Part model, mm, in its own coordinate system. Face numbers are marked on the shaded views. A direction names the side the tool comes from. Round coordinates to 2 decimals unless told otherwise and drop trailing zeros. Write each loop counter-clockwise with the first axis right and the second up, starting at its lowest first coordinate (ties: lowest second). Pieces come first, ordered by that corner, then holes. Notation, with made-up numbers: M -30.5,-37.75 L -10.5,-37.75 A22 cw -10.5,-30.75 Z; hole C 40.5,67.5 d1. An arc over 180 degrees is marked long. One line per question, with ' | ' between items. Start each with the question number.
1) Saw through at B-B (x = 0). Give the number of separate pieces and of enclosed holes in the cut face, plus the area to 3 significant figures.
2) Saw through at D-D (z = 42). List the corners of the cut face in (x, y), plus the area to 3 significant figures.
3) Saw through at A-A (y = 0). List the corners of the cut face in (x, z).
4) Saw through at C-C (z = 53). List the corners of the cut face in (x, y), plus the area to 3 significant figures.
5) Wall check: probe 1 along X at (y, z) = (-28.5, 4.5); probe 2 along X at (y, z) = (-46, 27); probe 3 along X at (y, z) = (-29, 16.5). Give the ranges that are in metal, low to high. Write a range as [from, to].
6) Mould opens along Y. For the marked faces 4, 5 and 6 say: pulls with the +Y half, pulls with the -Y half, needs draft (parallel to the pull), parting line crosses it, or undercut.
7) Tool access for the marked faces 1, 2 and 3: list every direction of +Z, -Z, +X, -X, +Y, -Y with a clear straight run to the whole face (end or side of a thin tool).
8) Drop flat-ended pins along their axis: pin 1 Ø10.5 at (x, y) = (53.5, -24.5) entering from +Z; pin 2 Ø10 at (y, z) = (57.5, 7) entering from +X; pin 3 Ø9 at (x, y) = (-55.42, -31.99) entering from +Z; pin 4 Ø10 at (y, z) = (24, 42.5) entering from +X. Give the stop position or say it passes through.
```python
from build123d import *

# Parameters (mm, degrees)
SKETCH1_R                    = 50
SKETCH1_R_2                  = 31.75
BOSS_EXTRUDE1_DEPTH          = 65
BOSS_EXTRUDE2_DEPTH          = 25
BOSS_EXTRUDE3_DEPTH          = 15
CHAMFER2_SIZE                = 2.5
F_10_0MM_DOWEL_HOLE1_D       = 10
CIRPATTERN2_COUNT            = 3
CHAMFER2_OF_CIRPATTERN2_SIZE = 2.5
CHAMFER1_SIZE                = 10
SKETCH2_R                    = 27.5
BOSS_EXTRUDE4_DEPTH          = 5
BOSS_EXTRUDE5_REACH          = 164.658
BOSS_EXTRUDE5_END_RADIUS     = 50
SKETCH3_R                    = 22.5
CUT_EXTRUDE1_REACH           = 168.801
CUT_EXTRUDE1_END_RADIUS      = 31.75
SKETCH4_R                    = 17.5


with BuildPart() as part:
    # Sketch1 → Boss-Extrude1 (new body)
    with BuildSketch(Plane.XY):
        Circle(SKETCH1_R)
        Circle(SKETCH1_R_2, mode=Mode.SUBTRACT)
    extrude(amount=BOSS_EXTRUDE1_DEPTH)

    # Sketch1<3> → Boss-Extrude2 (add)
    with BuildSketch(Plane.XY):
        with BuildLine():
            Line((-5, 20.603827518), (0, 20.603827518))
            Line((0, 20.603827518), (0, 31.75))
            ThreePointArc((0, 31.75), (-2.507835353, 31.650801915), (-5, 31.353827518))
            Line((-5, 31.353827518), (-5, 20.603827518))
        make_face()
        with BuildLine():
            Line((0, 31.75), (0, 20.603827518))
            Line((0, 20.603827518), (5, 20.603827518))
            Line((5, 20.603827518), (5, 31.353827518))
            ThreePointArc((5, 31.353827518), (2.507835353, 31.650801915), (0, 31.75))
        make_face()
    extrude(amount=BOSS_EXTRUDE2_DEPTH)

    # Sketch1<4> → Boss-Extrude3 (add)
    with BuildSketch(Plane.XY):
        with BuildLine():
            Line((-10, 63.989794856), (-10, 48.989794856))
            ThreePointArc((-10, 48.989794856), (0, 50), (10, 48.989794856))
            Line((10, 48.989794856), (10, 63.989794856))
            ThreePointArc((10, 63.989794856), (0, 73.989794856), (-10, 63.989794856))
        make_face()
    boss_extrude3 = extrude(amount=BOSS_EXTRUDE3_DEPTH)

    # Chamfer2
    chamfer2_edges = [part.edges().sort_by_distance(p)[0] for p in [
        (0, 73.989794856, 15),
        (-10, 56.489794856, 15),
        (10, 56.489794856, 15),
    ]]
    chamfer(chamfer2_edges, length=CHAMFER2_SIZE)

    # Ø10.0mm Dowel Hole1 (through all)
    with Locations(Plane.XY.offset(15)):
        with Locations((0, 63.989794856)):
            f_10_0mm_dowel_hole1 = Hole(F_10_0MM_DOWEL_HOLE1_D / 2)

    # CirPattern2: Boss-Extrude3, Ø10.0mm Dowel Hole1 ×3 about axis
    cirpattern2_axis = Axis((0, 0, 0), (0, 0, 1))
    add([boss_extrude3.rotate(cirpattern2_axis, i * 360 / CIRPATTERN2_COUNT) for i in range(1, CIRPATTERN2_COUNT)])
    add([f_10_0mm_dowel_hole1.rotate(cirpattern2_axis, i * 360 / CIRPATTERN2_COUNT) for i in range(1, CIRPATTERN2_COUNT)], mode=Mode.SUBTRACT)

    # Chamfer2 of CirPattern2
    chamfer2_of_cirpattern2_edges = [part.edges().sort_by_distance(p)[0] for p in [
        (-64.077041966, -36.994897428, 15),
        (-43.9215974, -36.905151466, 15),
        (-53.9215974, -19.58464339, 15),
        (64.077041966, -36.994897428, 15),
        (53.9215974, -19.58464339, 15),
        (43.9215974, -36.905151466, 15),
    ]]
    chamfer(chamfer2_of_cirpattern2_edges, length=CHAMFER2_OF_CIRPATTERN2_SIZE)

    # Chamfer1
    chamfer1_edges = [part.edges().sort_by_distance(p)[0] for p in [
        (-50, 0, 65),
    ]]
    chamfer(chamfer1_edges, length=CHAMFER1_SIZE)



with BuildPart() as body_2:
    # Sketch2 → Boss-Extrude4 (new body)
    with BuildSketch(Plane(origin=(0, -65, 0), x_dir=(1, 0, 0), z_dir=(0, 1, 0))):
        with Locations(Location((0, -27.5, 0), (0, 0, 270))):
            Circle(SKETCH2_R)
    extrude(amount=BOSS_EXTRUDE4_DEPTH)


with BuildPart() as part_1:
    add(part.part)

    add(body_2.part)  # Boss-Extrude5 merges body 2
    # Boss-Extrude5: up to this cylinder (the profile starts outside it)
    boss_extrude5_end = Plane(origin=(0, 0, 27.5), z_dir=(0, 0, -1)) * Cylinder(BOSS_EXTRUDE5_END_RADIUS, 430.316, mode=Mode.PRIVATE)
    # Sketch3 → Boss-Extrude5 (add, up to the surface)
    with BuildSketch(Plane(origin=(0, -60, 0), x_dir=(1, 0, 0), z_dir=(0, 1, 0)), mode=Mode.PRIVATE) as boss_extrude5_sk1:
        with Locations(Location((0, -27.5, 0), (0, 0, 90))):
            Circle(SKETCH3_R)
    boss_extrude5_tool1 = extrude(boss_extrude5_sk1.sketch, amount=BOSS_EXTRUDE5_REACH, mode=Mode.PRIVATE) - boss_extrude5_end
    add(boss_extrude5_tool1.solids().sort_by_distance((0, -60, 27.5))[0])

    # Cut-Extrude1: up to this cylinder (the profile starts outside it)
    cut_extrude1_end = Plane(origin=(0, 0, 27.5), z_dir=(0, 0, -1)) * Cylinder(CUT_EXTRUDE1_END_RADIUS, 402.102, mode=Mode.PRIVATE)
    # Sketch4 → Cut-Extrude1 (cut, up to the surface)
    with BuildSketch(Plane.XZ.offset(65), mode=Mode.PRIVATE) as cut_extrude1_sk1:
        with Locations(Location((0, 27.5, 0), (0, 0, 270))):
            Circle(SKETCH4_R)
    cut_extrude1_tool1 = extrude(cut_extrude1_sk1.sketch, amount=-CUT_EXTRUDE1_REACH, mode=Mode.PRIVATE) - cut_extrude1_end
    add(cut_extrude1_tool1.solids().sort_by_distance((0, -65, 27.5))[0], mode=Mode.SUBTRACT)


solid = part_1.part
```
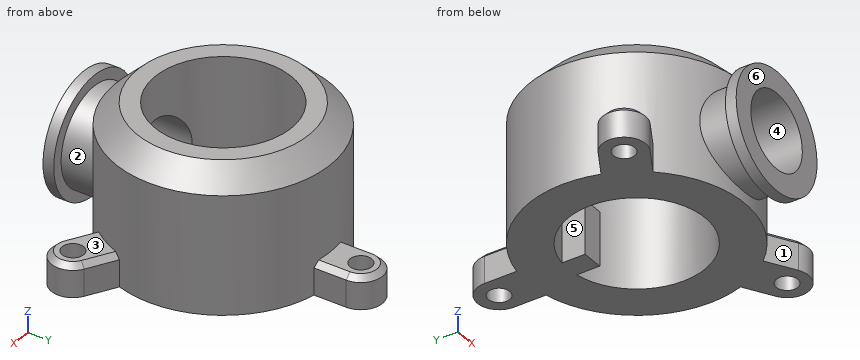
Answer key:
1) separate pieces: 4 | enclosed holes: 0 | area: 2,320 mm2
2) outline: M -23.37,-65 L -9.8,-65 L -9.8,-30.2 A31.75 cw long 9.8,-30.2 L 9.8,-65 L 23.37,-65 L 23.37,-60 L 17.2,-60 L 17.2,-46.95 A50 ccw long -17.2,-46.95 L -17.2,-60 L -23.37,-60 Z | area: 4,640 mm2
3) outline: M -50,0 L -31.75,0 L -31.75,65 L -40,65 L -50,55 Z; M 31.75,0 L 50,0 L 50,55 L 40,65 L 31.75,65 Z
4) outline: C 0,0 d100; M -10.3,-65 L 10.3,-65 L 10.3,-60 L -10.3,-60 Z; hole C 0,0 d63.5 | area: 4,790 mm2
5) probe 1: x = [-64.79, -58.99], [-51.84, -13.99], [13.99, 51.84], [58.99, 64.79] | probe 2: x = [-22.49, -17.49], [17.49, 22.49] | probe 3: x = [-40.73, -13.61], [13.61, 40.73]
6) face 4: needs draft | face 5: undercut | face 6: pulls with the -Y half
7) face 1: +Z, -Z, -Y | face 2: none | face 3: +Z, +X, -Y
8) pin 1: stops at z = 15 | pin 2: stops at x = 10 | pin 3: passes through | pin 4: stops at x = 46.25
